Source: CAD feature listing. Evaluate the final solid. Frame: model axes, mm. Round coordinates to 2 decimals unless told otherwise and drop trailing zeros. Loops run counter-clockwise (first coordinate to the right, second up) from the corner with the lowest first, then second, coordinate; pieces in that order, holes last.
(1) Section D-D, the plane x = -4. Return the cut outline in (y, z) (3 decimals), plus the area to 3 significant figures.
(2) Section B-B, the plane x = 0. Return the cut outline in (y, z) (3 decimals), plus the area to 3 significant figures.
(3) Section A-A, the plane y = 1.8. Return the cut outline in (x, z) (3 decimals).
(4) Section C-C, the plane z = 0. Return the cut outline in (x, y) (3 decimals), plus the area to 3 significant figures.
(5) First-contact query: pin 1 Ø3 at (x, z) = (0, 16.5) entering from +Y. Flat tip, straight axial feed; report the tip coordinate or a pass-through.
(6) Material intervals for probe 1 along Z at (x, y) = (0, 2.5); probe 2 along Z at (x, y) = (1, 2.3); probe 3 along Z at (x, y) = (-13.5, 2), sorted ascending.
(7) Mould query, pull axis Z, two halves, no side actions, for faces 1 (the cylindrical face through (15.959, 1.565, -8.776)), 2 (the flat face through (0, 3.175, -7)), 3 (the flat face through (9.86, 1.57, 5.92)), 4 (the cylindrical face through (-17.08, 1.565, -9.916)). Classes: pulls with the +Z half, pulls with the -Z half, needs draft (parallel to the pull), parting line crosses it, or undercut.
```python
from build123d import *

# Parameters (mm, degrees)
SKETCH1_R           = 5.334
SKETCH1_R_2         = 1.75
BOSS_EXTRUDE1_DEPTH = 3.175


with BuildPart() as part:
    # Sketch1 → Boss-Extrude1 (new body)
    with BuildSketch(Plane(origin=(0, 0, 0), x_dir=(1, 0, 0), z_dir=(0, 1, 0))):
        with BuildLine():
            Line((-17.104001725, 6.625), (-2.814582562, -18.125))
            ThreePointArc((-2.814582562, -18.125), (0, -19.75), (2.814582562, -18.125))
            Line((2.814582562, -18.125), (17.104001725, 6.625))
            ThreePointArc((17.104001725, 6.625), (17.104001725, 9.875), (14.289419162, 11.5))
            Line((14.289419162, 11.5), (-14.289419162, 11.5))
            ThreePointArc((-14.289419162, 11.5), (-17.104001725, 9.875), (-17.104001725, 6.625))
        make_face()
        Circle(SKETCH1_R, mode=Mode.SUBTRACT)
        with Locations((-14.289419162, 8.25)):
            Circle(SKETCH1_R_2, mode=Mode.SUBTRACT)
        with Locations((0, -16.5)):
            Circle(SKETCH1_R_2, mode=Mode.SUBTRACT)
        with Locations((14.289419162, 8.25)):
            Circle(SKETCH1_R_2, mode=Mode.SUBTRACT)
    extrude(amount=BOSS_EXTRUDE1_DEPTH)


solid = part.part
```
Output values:
1. outline: (0, -11.5) - (3.175, -11.5) - (3.175, -3.529) - (0, -3.529) - close; (0, 3.529) - (3.175, 3.529) - (3.175, 16.072) - (0, 16.072) - close
1. area: 65.1 mm2
2. outline: (0, -11.5) - (3.175, -11.5) - (3.175, -5.334) - (0, -5.334) - close; (0, 5.334) - (3.175, 5.334) - (3.175, 14.75) - (0, 14.75) - close; (0, 18.25) - (3.175, 18.25) - (3.175, 19.75) - (0, 19.75) - close
2. area: 54.2 mm2
3. outline: (-17.104, -6.625) arc R3.25 ccw to (-14.289, -11.5) - (14.289, -11.5) arc R3.25 ccw to (17.104, -6.625) - (2.815, 18.125) arc R3.25 ccw to (-2.815, 18.125) - close; hole circle Ø3.5 at (-14.289, -8.25); hole circle Ø10.668 at (0, 0); hole circle Ø3.5 at (0, 16.5); hole circle Ø3.5 at (14.289, -8.25)
4. outline: (-13.279, 0) - (-5.334, 0) - (-5.334, 3.175) - (-13.279, 3.175) - close; (5.334, 0) - (13.279, 0) - (13.279, 3.175) - (5.334, 3.175) - close
4. area: 50.5 mm2
5. pin 1: passes through
6. probe 1: z = -11.5 to -5.33, 5.33 to 14.75, 18.25 to 19.75
6. probe 2: z = -11.5 to -5.24, 5.24 to 15.06, 17.94 to 19.59
6. probe 3: z = -11.5 to -9.81, -6.69 to -0.38
7. face 1: undercut
7. face 2: needs draft
7. face 3: pulls with the +Z half
7. face 4: parting line crosses it
